The listing builds one solid part. Answer for the finished solid, in the listing's coordinates (mm). Coordinates: 2 decimals unless noted, no trailing zeros. Loops run counter-clockwise (first coordinate to the right, second up) from the corner with the lowest first, then second, coordinate; pieces in that order, holes last. Notation, with made-up numbers: (-21.5, 41.25) - (28.5, 41.25) arc R31 cw to (28.5, 78.25) - close; hole circle Ø11 at (12.5, 22.25). An arc over 180 degrees is marked (long way). Return JSON: item names as keys, results as strings. Group by question number.
1. Section C-C (y = 5.75) is taken. Write down the section's boundary in (x, z).
2. Section B-B (x = 3.5) is taken. Write down the section's boundary in (y, z), and give its area (3 significant figures).
3. Section A-A (y = 13.5) is taken. Write down the section's boundary in (x, z) (3 decimals), and give its area (3 significant figures).
4. Section D-D (z = 1.1) is taken. Write down the section's boundary in (x, y) (3 decimals), and give its area (3 significant figures).
5. Each of these flat-tipped pins is pushed along its axis until it touches: P1, Ø1, axis at y = 7.5, z = 1.5, coming from the -X side; P2, Ø1, axis at y = 6.5, z = 1, coming from the +X side. Where does it stop, or does it pass through?
6. Find the intervals of material crossed by line 1 along Y through (x, z) = (-1, 0.3); line 2 along Y through (x, z) = (-5.25, 1); line 3 along X through (y, z) = (22, 0.2), in increasing order.
```python
from build123d import *

# Parameters (mm, degrees)
SKETCH1_R           = 1.06
BOSS_EXTRUDE1_DEPTH = 2


with BuildPart() as part:
    # Sketch1 → Boss-Extrude1 (new body)
    with BuildSketch(Plane.XY):
        with BuildLine():
            Line((-9.06, 28.183587826), (9.06, 28.183587826))
            ThreePointArc((9.06, 28.183587826), (10.474213562, 27.597801388), (11.06, 26.183587826))
            Line((11.06, 26.183587826), (11.06, 16.909233785))
            ThreePointArc((11.06, 16.909233785), (13.735, 13.5), (11.06, 10.090766215))
            Line((11.06, 10.090766215), (11.06, 0.816412174))
            ThreePointArc((11.06, 0.816412174), (10.474213562, -0.597801388), (9.06, -1.183587826))
            Line((9.06, -1.183587826), (-9.06, -1.183587826))
            ThreePointArc((-9.06, -1.183587826), (-10.474213562, -0.597801388), (-11.06, 0.816412174))
            Line((-11.06, 0.816412174), (-11.06, 10.090766215))
            ThreePointArc((-11.06, 10.090766215), (-13.735, 13.5), (-11.06, 16.909233785))
            Line((-11.06, 16.909233785), (-11.06, 26.183587826))
            ThreePointArc((-11.06, 26.183587826), (-10.474213562, 27.597801388), (-9.06, 28.183587826))
        make_face()
        with Locations((-10.225, 13.5)):
            Circle(SKETCH1_R, mode=Mode.SUBTRACT)
        with Locations((10.225, 13.5)):
            Circle(SKETCH1_R, mode=Mode.SUBTRACT)
        with BuildLine():
            Line((-5, 4.9), (5, 4.9))
            ThreePointArc((5, 4.9), (5.353553391, 5.046446609), (5.5, 5.4))
            Line((5.5, 5.4), (5.5, 9.4))
            ThreePointArc((5.5, 9.4), (5.353553391, 9.753553391), (5, 9.9))
            Line((5, 9.9), (-5, 9.9))
            ThreePointArc((-5, 9.9), (-5.353553391, 9.753553391), (-5.5, 9.4))
            Line((-5.5, 9.4), (-5.5, 5.4))
            ThreePointArc((-5.5, 5.4), (-5.353553391, 5.046446609), (-5, 4.9))
        make_face(mode=Mode.SUBTRACT)
    extrude(amount=BOSS_EXTRUDE1_DEPTH)


solid = part.part
```
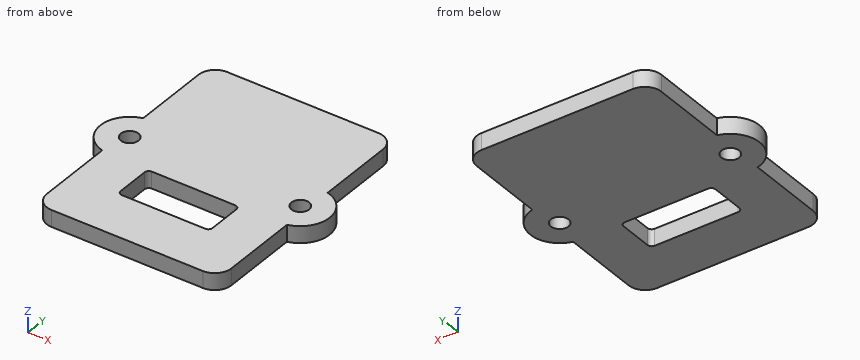
The answers:
{
 "1": {"outline": "(-11.06, 0) - (-5.5, 0) - (-5.5, 2) - (-11.06, 2) - close; (5.5, 0) - (11.06, 0) - (11.06, 2) - (5.5, 2) - close"},
 "2": {"outline": "(-1.18, 0) - (4.9, 0) - (4.9, 2) - (-1.18, 2) - close; (9.9, 0) - (28.18, 0) - (28.18, 2) - (9.9, 2) - close", "area": "48.7 mm2"},
 "3": {"outline": "(-13.735, 0) - (-11.285, 0) - (-11.285, 2) - (-13.735, 2) - close; (-9.165, 0) - (9.165, 0) - (9.165, 2) - (-9.165, 2) - close; (11.285, 0) - (13.735, 0) - (13.735, 2) - (11.285, 2) - close", "area": "46.5 mm2"},
 "4": {"outline": "(-11.06, 0.816) arc R2 ccw to (-9.06, -1.184) - (9.06, -1.184) arc R2 ccw to (11.06, 0.816) - (11.06, 10.091) arc R3.51 ccw to (11.06, 16.909) - (11.06, 26.184) arc R2 ccw to (9.06, 28.184) - (-9.06, 28.184) arc R2 ccw to (-11.06, 26.184) - (-11.06, 16.909) arc R3.51 ccw to (-11.06, 10.091) - close; hole circle Ø2.12 at (-10.225, 13.5); hole (-5.5, 5.4) arc R0.5 ccw to (-5, 4.9) - (5, 4.9) arc R0.5 ccw to (5.5, 5.4) - (5.5, 9.4) arc R0.5 ccw to (5, 9.9) - (-5, 9.9) arc R0.5 ccw to (-5.5, 9.4) - close; hole circle Ø2.12 at (10.225, 13.5)", "area": "611 mm2"},
 "5": {"P1": "stops at x = -11.06", "P2": "stops at x = 11.06"},
 "6": {"line 1": "y = -1.18 to 4.9, 9.9 to 28.18", "line 2": "y = -1.18 to 4.97, 9.83 to 28.18", "line 3": "x = -11.06 to 11.06"}
}
